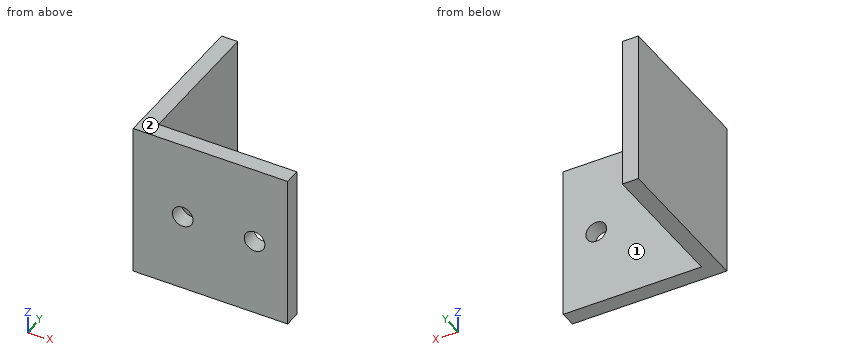
```python
from build123d import *

# Parameters (mm, degrees)
EXTRUS_O_FINA1_DEPTH  = 30
ESBO_O2_R             = 2
CORTE_EXTRUS_O1_DEPTH = 30


with BuildPart() as part:
    # Esboço1 → Extrusão-Fina1 (new body)
    with BuildSketch(Plane.XY):
        Polygon((0, 0), (-30, 0), (-30, 30), (-26.875, 30), (-26.875, 3.125), (0, 3.125), align=None)
    extrude(amount=EXTRUS_O_FINA1_DEPTH)

    # Esboço2 → Corte-extrusão1 (cut)
    with BuildSketch(Plane(origin=(0, 3.125, 0), x_dir=(1, 0, 0), z_dir=(0, 1, 0))):
        with Locations(Location((-6.417692874, -15, 0), (0, 0, 180))):  # turned: the seam where the file's is
            Circle(ESBO_O2_R)
        with Locations(Location((-20.380879672, -15, 0), (0, 0, 180))):  # turned: the seam where the file's is
            Circle(ESBO_O2_R)
    extrude(amount=-CORTE_EXTRUS_O1_DEPTH, mode=Mode.SUBTRACT)


solid = part.part
```
Can you work these out from the model? Positions are in its coordinate system, mm. Face numbers are marked on the shaded views. A direction names the side the tool comes from. Coordinates: 2 decimals unless noted, no trailing zeros. Loops run counter-clockwise (first coordinate to the right, second up) from the corner with the lowest first, then second, coordinate; pieces in that order, holes last. Notation, with made-up numbers: (29.5, 38.25) - (59.5, 38.25) arc R17 ccw to (59.5, 49.25) - close; hole circle Ø11 at (-21, 21). An arc over 180 degrees is marked (long way). Answer as CSV lines item,"result". Start each with the question number.
1) Which directions (+Z, -Z, +X, -X, +Y, -Y) give clear straight access to the entire face, cutting with the end or side of a thin tool? Please do the marked faces 1 and 2.
2) Suppose I cut it at B-B (x = -19). Please give me the cut outline in (y, z) (3 decimals).
3) Suppose I cut it at D-D (x = -10.25). Please give me the cut outline in (y, z) (3 decimals), plus the area to 4 significant figures.
4) Suppose I cut it at C-C (z = 7). Please give me the cut outline in (x, y) (3 decimals).
5) I need wall thicknesses on line 1 (Y direction, x = -17.5, z = 7.5) (3 decimals); line 2 (X direction, y = 23.5, z = 21.25) (3 decimals). Which ranges of each line are inside material? Lowest first, please. Write a range as from..to.
6) Suppose I cut it at A-A (z = 15). Please give me the cut outline in (x, y) (3 decimals), plus the area to 3 significant figures.
7) For pin 1 (8 mm diameter, centred on y = 11, z = 22.5, fed in from +X) (3 decimals); pin 2 (4.5 mm diameter, centred on x = -20.38, z = 15, fed in from +Y) (3 decimals), each with a flat end and sliding along its axis, tell me the tip position at first contact or that it passes through.
Check result:
1,face 1,"+Z, -Z, +X, +Y"
1,face 2,"+Z, +X, -X, +Y, -Y"
2,outline,"(0, 0) - (3.125, 0) - (3.125, 13.553) - (0, 13.553) - close; (0, 16.447) - (3.125, 16.447) - (3.125, 30) - (0, 30) - close"
3,outline,"(0, 0) - (3.125, 0) - (3.125, 30) - (0, 30) - close"
3,area,"93.75 mm²"
4,outline,"(-30, 0) - (0, 0) - (0, 3.125) - (-26.875, 3.125) - (-26.875, 30) - (-30, 30) - close"
5,line 1,"y = 0..3.125"
5,line 2,"x = -30..-26.875"
6,outline,"(-30, 0) - (-22.381, 0) - (-22.381, 3.125) - (-26.875, 3.125) - (-26.875, 30) - (-30, 30) - close; (-18.381, 0) - (-8.418, 0) - (-8.418, 3.125) - (-18.381, 3.125) - close; (-4.418, 0) - (0, 0) - (0, 3.125) - (-4.418, 3.125) - close"
6,area,"153 mm²"
7,pin 1,"stops at x = -26.875"
7,pin 2,"stops at y = 3.125"
